from build123d import *

# Parameters (mm, degrees)
EXTRUDE_1_DEPTH     = 3
EXTRUDE_1_2_DEPTH   = 0.3
EXTRUDE_START       = 2.5
EXTRUDE_2_DEPTH     = 2.5
CUT_EXTRUDE_1_DEPTH = 4.52
EXTRUDE_START_2     = 4
EXTRUDE_2_2_DEPTH   = 4
SKETCH_6_W          = 13.6
SKETCH_6_H          = 0.2
CUT_EXTRUDE_2_DEPTH = 3


with BuildPart() as part:
    # Эскиз1 → Extrude 1 (new body)
    with BuildSketch(Plane(origin=(0, 0, 0), x_dir=(1, 0, 0), z_dir=(0, 1, 0))):
        with BuildLine():
            Line((13.6, -3.06), (0, -3.06))
            ThreePointArc((0, -3.06), (-3.06, 0), (0, 3.06))
            Line((0, 3.06), (13.6, 3.06))
            ThreePointArc((13.6, 3.06), (16.66, 0), (13.6, -3.06))
        make_face()
        with BuildLine():
            Line((13.6, -2.26), (0, -2.26))
            ThreePointArc((0, -2.26), (-2.26, 0), (0, 2.26))
            Line((0, 2.26), (13.6, 2.26))
            ThreePointArc((13.6, 2.26), (15.86, 0), (13.6, -2.26))
        make_face(mode=Mode.SUBTRACT)
    extrude(amount=EXTRUDE_1_DEPTH)

    # Эскиз2 → Extrude 1 2 (add)
    with BuildSketch(Plane(origin=(0, 3, 0), x_dir=(1, 0, 0), z_dir=(0, 1, 0))):
        with BuildLine():
            Line((0, 3.5), (13.6, 3.5))
            ThreePointArc((13.6, 3.5), (17.1, 0), (13.6, -3.5))
            Line((13.6, -3.5), (0, -3.5))
            ThreePointArc((0, -3.5), (-3.5, 0), (0, 3.5))
        make_face()
    extrude(amount=EXTRUDE_1_2_DEPTH)

    # Эскиз3 → Extrude 2 (add)
    with BuildSketch(Plane.XZ.offset(-3).offset(EXTRUDE_START)):
        with BuildLine():
            Line((0, -2.26), (2, -2.26))
            Line((2, -2.26), (2, 2.26))
            Line((2, 2.26), (0, 2.26))
            ThreePointArc((0, 2.26), (-2.26, 0), (0, -2.26))
        make_face()
    extrude(amount=-EXTRUDE_2_DEPTH)

    # Эскиз4 → Вырез-Вытянуть1 (cut)
    with BuildSketch(Plane.XY.offset(-2.26)):
        Polygon((2, 3), (0.2, 3), (2, 1.2), align=None)
    extrude(amount=CUT_EXTRUDE_1_DEPTH, mode=Mode.SUBTRACT)

    # Эскиз5 → Extrude 2 2 (add)
    with BuildSketch(Plane.XZ.offset(EXTRUDE_START_2)):
        with BuildLine():
            ThreePointArc((13.6, -2.26), (15.86, 0), (13.6, 2.26))
            Line((13.6, 2.26), (13.6, 3.06))
            ThreePointArc((13.6, 3.06), (16.66, 0), (13.6, -3.06))
            Line((13.6, -3.06), (13.6, -2.26))
        make_face()
    extrude(amount=-EXTRUDE_2_2_DEPTH)

    # Эскиз6 → Вырез-Вытянуть2 (cut)
    with BuildSketch(Plane.XZ):
        with Locations((6.8, 2.96)):
            Rectangle(SKETCH_6_W, SKETCH_6_H)
        with Locations((6.8, -2.96)):
            Rectangle(SKETCH_6_W, SKETCH_6_H)
    extrude(amount=-CUT_EXTRUDE_2_DEPTH, mode=Mode.SUBTRACT)


solid = part.part
Can you work these out from the model? Positions are in its coordinate system, mm. A direction names the side the tool comes from. Coordinates: 2 decimals unless noted, no trailing zeros. Write each loop counter-clockwise with the first axis right and the second up, starting at its lowest first coordinate (ties: lowest second). Pieces come first, ordered by that corner, then holes.
Q1. Please list where these lines run through material, in increasing order: L1, parallel to Z at x = 2.5, y = 1.25; L2, parallel to Y at x = 0, z = -0.75; L3, parallel to X at y = -1, z = 0.
Results found:
L1: z = -2.86 to -2.26, 2.26 to 2.86
L2: y = 0.5 to 3.3
L3: x = 15.86 to 16.66
Q2. Imagine slicing it at D-D, the plane x = 1.75. List the corners of the cut face in (y, z) for me, plus the area to 3 significant figures.
Results found:
outline: (0, -2.86) - (3, -2.86) - (3, -3.5) - (3.3, -3.5) - (3.3, 3.5) - (3, 3.5) - (3, 2.86) - (0, 2.86) - (0, 2.26) - (0.5, 2.26) - (0.5, -2.26) - (0, -2.26) - close; hole (1.45, -2.26) - (3, -2.26) - (3, 2.26) - (1.45, 2.26) - close
area: 9.99 mm2
Q3. Imagine slicing it at B-B, the plane z = 0. List the corners of the cut face in (x, y) for me, plus the area to 3 significant figures.
Results found:
outline: (-3.5, 3) - (-3.06, 3) - (-3.06, 0) - (-2.26, 0) - (-2.26, 0.5) - (2, 0.5) - (2, 1.2) - (0.2, 3) - (15.86, 3) - (15.86, -4) - (16.66, -4) - (16.66, 3) - (17.1, 3) - (17.1, 3.3) - (-3.5, 3.3) - close
area: 23.2 mm2
Q4. Imagine slicing it at C-C, the plane x = 8.5. List the corners of the cut face in (y, z) for me, plus the area to 3 significant figures.
Results found:
outline: (0, -2.86) - (3, -2.86) - (3, -3.5) - (3.3, -3.5) - (3.3, 3.5) - (3, 3.5) - (3, 2.86) - (0, 2.86) - (0, 2.26) - (3, 2.26) - (3, -2.26) - (0, -2.26) - close
area: 5.70 mm2
Q5. Imagine slicing it at A-A, the plane y = 0.75. List the corners of the cut face in (x, z) for me.
Results found:
outline: (0, -3.06) - (0, -2.86) - (13.6, -2.86) - (13.6, -3.06) arc R3.06 ccw to (13.6, 3.06) - (13.6, 2.86) - (0, 2.86) - (0, 3.06) arc R3.06 ccw to start; hole (2, -2.26) - (13.6, -2.26) arc R2.26 ccw to (13.6, 2.26) - (2, 2.26) - close
Q6. For P1, Ø3.5, axis at x = 4, z = 1, coming from the -Y side; P2, Ø4, axis at y = 0, z = -2, coming from the +X side; P3, Ø3, axis at x = 14.5, y = 2.5, coming from the -Z side; P4, Ø3.5, axis at x = 5.5, y = 1, coming from the +Z side, each with a flat end and sliding along its axis, tell me the tip position at first contact or that it passes through.
Results found:
P1: stops at y = 0
P2: stops at x = 16.66
P3: stops at z = -3.5
P4: stops at z = 2.86
Q7. Which directions (+Z, -Z, +X, -X, +Y, -Y) give clear straight access to the entire face, cutting with the end or side of a thin tool? Please do faces 5 (the face through (-3.06, 1.48, 0.07)), 6 (the face through (15.86, -0.55, -0.05)), 7 (the face through (7, 1, -2.86)), 8 (the face through (13.6, -1.3, 2.7)).
Results found:
face 5: -X, -Y
face 6: -Y
face 7: -Z, -Y
face 8: +Z, -Y
Q8. If we mould it in two halves opening along X, with no side actions, what happens to faces 1 (the face through (-2.26, 0.25, 0.05)), 2 (the face through (17.1, 3.15, -0.08)), 3 (the face through (5.3, 0, -2.5)), 4 (the face through (0, 0.5, 0))? For each: +X half, -X half, draft (parallel to the pull), parting line (faces both ways), or undercut.
Results found:
face 1: undercut
face 2: +X half
face 3: draft
face 4: undercut
